from build123d import *

# Parameters (mm, degrees)
SKETCH1_R                       = 12.7
BOSS_EXTRUDE1_DEPTH             = 30.1625
SKETCH4_R                       = 15.875
BOSS_EXTRUDE2_DEPTH             = 50.8
CUT_EXTRUDE1_DEPTH              = 11.176
SKETCH3_R                       = 6
CUT_EXTRUDE2_DEPTH              = 8
SKETCH5_R                       = 3.175
BOSS_EXTRUDE3_DEPTH             = 6.604
F_8_32_TAPPED_HOLE1_D           = 3.4544
CUT_EXTRUDE3_START              = -6.35
SKETCH9_R                       = 15.875
SKETCH9_R_2                     = 6.35
CUT_EXTRUDE3_DEPTH              = 38.1
FILLET1_R                       = 3.175
CHAMFER1_SIZE                   = 1.27
F_1_4_0_25_DIAMETER_HOLE1_D     = 6.35
F_1_4_0_25_DIAMETER_HOLE1_DEPTH = 6.35
F_1_4_0_25_DIAMETER_HOLE1_TIP   = 1.907732465
CHAMFER2_SIZE                   = 0.762


with BuildPart() as part:
    # Sketch1 → Boss-Extrude1 (new body)
    with BuildSketch(Plane(origin=(0, 0, 0), x_dir=(1, 0, 0), z_dir=(0, 1, 0))):
        Circle(SKETCH1_R)
    extrude(amount=BOSS_EXTRUDE1_DEPTH)

    # Sketch4 → Boss-Extrude2 (add)
    with BuildSketch(Plane(origin=(0, 30.1625, 0), x_dir=(1, 0, 0), z_dir=(0, 1, 0))):
        Circle(SKETCH4_R)
    extrude(amount=BOSS_EXTRUDE2_DEPTH)

    # Sketch2 → Cut-Extrude1 (cut)
    with BuildSketch(Plane.XZ):
        with BuildLine():
            Line((-7, 2.899494937), (-8.776962921, 1.122532015))
            ThreePointArc((-8.776962921, 1.122532015), (-9.241930906, 0), (-8.776962921, -1.122532015))
            Line((-8.776962921, -1.122532015), (-7, -2.899494937))
            Line((-7, -2.899494937), (-7, 2.899494937))
        make_face()
        Polygon((-2.899494937, 7), (-7, 2.899494937), (-7, -2.899494937), (-2.899494937, -7), (2.899494937, -7), (7, -2.899494937), (7, 2.899494937), (2.899494937, 7), align=None)
        with BuildLine():
            Line((-7, 5.4125), (-7, 2.899494937))
            Line((-7, 2.899494937), (-2.899494937, 7))
            Line((-2.899494937, 7), (-5.4125, 7))
            ThreePointArc((-5.4125, 7), (-6.535032015, 6.535032015), (-7, 5.4125))
        make_face()
        with BuildLine():
            Line((-1.122532015, 8.776962921), (-2.899494937, 7))
            Line((-2.899494937, 7), (2.899494937, 7))
            Line((2.899494937, 7), (1.122532015, 8.776962921))
            ThreePointArc((1.122532015, 8.776962921), (0, 9.241930906), (-1.122532015, 8.776962921))
        make_face()
        with BuildLine():
            Line((5.4125, 7), (2.899494937, 7))
            Line((2.899494937, 7), (7, 2.899494937))
            Line((7, 2.899494937), (7, 5.4125))
            ThreePointArc((7, 5.4125), (6.535032015, 6.535032015), (5.4125, 7))
        make_face()
        with BuildLine():
            Line((8.776962921, 1.122532015), (7, 2.899494937))
            Line((7, 2.899494937), (7, -2.899494937))
            Line((7, -2.899494937), (8.776962921, -1.122532015))
            ThreePointArc((8.776962921, -1.122532015), (9.241930906, 0), (8.776962921, 1.122532015))
        make_face()
        with BuildLine():
            Line((7, -2.899494937), (2.899494937, -7))
            Line((2.899494937, -7), (5.4125, -7))
            ThreePointArc((5.4125, -7), (6.535032015, -6.535032015), (7, -5.4125))
            Line((7, -5.4125), (7, -2.899494937))
        make_face()
        with BuildLine():
            Line((2.899494937, -7), (-2.899494937, -7))
            Line((-2.899494937, -7), (-1.122532015, -8.776962921))
            ThreePointArc((-1.122532015, -8.776962921), (0, -9.241930906), (1.122532015, -8.776962921))
            Line((1.122532015, -8.776962921), (2.899494937, -7))
        make_face()
        with BuildLine():
            Line((-2.899494937, -7), (-7, -2.899494937))
            Line((-7, -2.899494937), (-7, -5.4125))
            ThreePointArc((-7, -5.4125), (-6.535032015, -6.535032015), (-5.4125, -7))
            Line((-5.4125, -7), (-2.899494937, -7))
        make_face()
    extrude(amount=-CUT_EXTRUDE1_DEPTH, mode=Mode.SUBTRACT)

    # Sketch3 → Cut-Extrude2 (cut)
    with BuildSketch(Plane.XZ.offset(-11.176)):
        Circle(SKETCH3_R)
    extrude(amount=-CUT_EXTRUDE2_DEPTH, mode=Mode.SUBTRACT)

    # Sketch5 → Boss-Extrude3 (add)
    with BuildSketch(Plane(origin=(0, 80.9625, 0), x_dir=(1, 0, 0), z_dir=(0, 1, 0))):
        Circle(SKETCH5_R)
    extrude(amount=BOSS_EXTRUDE3_DEPTH)

    # #8-32 Tapped Hole1 (through all)
    with Locations(Plane(origin=(0, 87.5665, 0), x_dir=(1, 0, 0), z_dir=(0, 1, 0))):
        with Locations((0, 0)):
            Hole(F_8_32_TAPPED_HOLE1_D / 2)

    # Sketch9 → Cut-Extrude3 (cut)
    with BuildSketch(Plane(origin=(0, 80.9625, 0), x_dir=(1, 0, 0), z_dir=(0, 1, 0)).offset(CUT_EXTRUDE3_START)):
        Circle(SKETCH9_R)
        Circle(SKETCH9_R_2, mode=Mode.SUBTRACT)
    extrude(amount=-CUT_EXTRUDE3_DEPTH, mode=Mode.SUBTRACT)

    # Fillet1
    fillet1_edges = [part.edges().sort_by_distance(p)[0] for p in [
        (-6.35, 36.5125, 0),
        (-6.35, 74.6125, 0),
    ]]
    fillet(fillet1_edges, radius=FILLET1_R)

    # Chamfer1
    chamfer1_edges = [part.edges().sort_by_distance(p)[0] for p in [
        (-15.875, 36.5125, 0),
    ]]
    chamfer(chamfer1_edges, length=CHAMFER1_SIZE)

    # Sketch10 → Cut-Revolve1 (revolve, cut)
    with BuildSketch(Plane.XY):
        Polygon((0, 87.5665), (0, 56.1975), (-6.3627, 56.1975), (-6.3627, 38.9382), (-15.875, 38.9382), (-15.875, 87.5665), align=None)
    revolve(axis=Axis((0, 87.5665, 0), (0, -1, 0)), mode=Mode.SUBTRACT)

    # 1/4 (0.25) Diameter Hole1
    with Locations(Plane(origin=(0, 56.1975, 0), x_dir=(1, 0, 0), z_dir=(0, 1, 0))):
        with Locations((0, 0)):
            Hole(F_1_4_0_25_DIAMETER_HOLE1_D / 2, depth=F_1_4_0_25_DIAMETER_HOLE1_DEPTH)
            with Locations((0, 0, -(F_1_4_0_25_DIAMETER_HOLE1_DEPTH + F_1_4_0_25_DIAMETER_HOLE1_TIP / 2))):  # 118° drill point
                Cone(0, F_1_4_0_25_DIAMETER_HOLE1_D / 2, F_1_4_0_25_DIAMETER_HOLE1_TIP, mode=Mode.SUBTRACT)

    # Chamfer2
    chamfer2_edges = [part.edges().sort_by_distance(p)[0] for p in [
        (-6.35, 56.1975, 0),
    ]]
    chamfer(chamfer2_edges, length=CHAMFER2_SIZE)


solid = part.part
Geometry: final body of the model. Coordinates: model frame, mm. A direction names the side the tool comes from. Give positions to 0.01 mm unless a question says otherwise; leave off trailing zeros. Write each loop counter-clockwise with the first axis right and the second up, starting at its lowest first coordinate (ties: lowest second). Pieces come first, ordered by that corner, then holes.
(1) First-contact query: P1, Ø2, axis at x = 10, z = -2, coming from the +Y side; P2, Ø3.5, axis at x = 1, z = 2, coming from the -Y side; P3, Ø1.3, axis at y = 6.5, z = -3.5, coming from the +X side. Flat tips, straight axial feed; report the tip coordinate or a pass-through.
(2) Cut plane B-B, the plane y = 13. Return loops of the section in (x, z).
(3) Access query for faces 4 (the flat face through (2.4, 56.198, 2.4)), 5 (the flat face through (-4, 6, -7)), 6 (the cylindrical face through (-1.38, 47.67, 6.2)). Directions: +Z, -Z, +X, -X, +Y, -Y. A direction counts if a zero-diameter tool reaches every point of the face in a straight line with its end or side. Return the directions, or none.
(4) Cut plane A-A, the plane y = 47. Return loops of the section in (x, z).
(5) Mould query, pull axis Z, two halves, no side actions, for faces 1 (the flat face through (4, 6, 7)), 2 (the cylindrical face through (-2.75, 14.87, 12.4)), 3 (the flat face through (-7, 30.162, -11)). Classes: released by +Z, released by -Z, zero draft, split by the parting line, or undercut.
(6) Ray query, line 1 (Z direction, x = 0, y = 15); line 2 (Z direction, x = 0, y = 33) (3 decimals); line 3 (X direction, y = 40, z = -5.5). Return the intervals inside material, ascending.
Values follow:
1. P1: stops at y = 36.53
1. P2: stops at y = 19.18
1. P3: stops at x = 12.38
2. outline: circle Ø25.4 at (0, 0); hole circle Ø12 at (0, 0)
3. face 4: +Z, -Z, +X, -X, +Y
3. face 5: -Y
3. face 6: +Y
4. outline: circle Ø12.7 at (0, 0); hole circle Ø3.45 at (0, 0)
5. face 1: undercut
5. face 2: split by the parting line
5. face 3: zero draft
6. line 1: z = -12.7 to -6, 6 to 12.7
6. line 2: z = -15.875 to -1.727, 1.727 to 15.875
6. line 3: x = -3.17 to 3.17
